Geometry: final body of the model. Coordinates: model frame, mm. A direction names the side the tool comes from. Coordinates: 2 decimals unless noted, no trailing zeros. Order: outer loops, then holes, each group sorted by start corner. A loop starts at its lowest first (then second) coordinate and runs counter-clockwise, first axis right, second up. Notation, with made-up numbers: (-18, 0) -> (32, 0) arc R29 cw to (32, 23) -> close; hole circle Ø10 at (9.5, 88). An arc over 180 degrees is marked (long way). Answer in a Markdown table with one row per item. Add a question column.
1) Section query A-A on x = 33. Return the cut outline in (y, z), then the cut area to 3 significant figures.
2) Section query B-B on y = 0. Return the cut outline in (x, z).
3) Set-up query: faces 4 (the face through (60.79, 13.61, 5.3)), 5 (the face through (-36.71, 28.26, 4.93)), 6 (the face through (-38.6, -1.9, 4.9)), 7 (the face through (-34.55, 8.38, 4.93)). Return all of +Z, -Z, +X, -X, +Y, -Y with unobstructed straight access to the full face (end or side cutting, diameter ignored); none if empty.
4) Ray query, line 1 (Y direction, x = 0, z = 7.75); line 2 (Y direction, x = 23.5, z = 0.5); line 3 (Y direction, x = -33.5, z = 1.75). Return the intervals inside material, ascending. Write a range as from..to.
5) Pull-direction query (Y, two-part tool) for faces 1 (the face through (-29.41, -92.26, 4.93)), 2 (the face through (11, -14, 0)), 3 (the face through (20.21, 23.37, 4.93)); classes: +Y half, -Y half, draft (parallel to the pull), parting line (faces both ways), or undercut.
6) Contact query for flat-ended pins moving along their axis: P1, Ø1.1, axis at x = 96, z = 7, coming from the -Y side; P2, Ø3, axis at y = -69, z = 6, coming from the +X side; P3, Ø3, axis at y = 17, z = 8, coming from the -X side. Output: stop coordinate, or through.
7) Section query D-D on z = 5.75. Count the separate pieces of the cut face and the enclosed holes in it, then the cut area to 3 significant figures.
8) Section query C-C on x = 0. Return the cut outline in (y, z).
```python
from build123d import *

# Parameters (mm, degrees)
SKETCH1_R           = 5.958520806
BOSS_EXTRUDE1_DEPTH = 10
SKETCH4_R           = 21.186821389
SKETCH4_R_2         = 2.5
CUT_EXTRUDE4_DEPTH  = 10
CUT_EXTRUDE5_DEPTH  = 24
SKETCH6_W           = 3.587503093
SKETCH6_H           = 10
CUT_EXTRUDE8_DEPTH  = 24
CUT_EXTRUDE9_DEPTH  = 24


with BuildPart() as part:
    # Sketch1 → Boss-Extrude1 (new body)
    with BuildSketch(Plane.XY):
        with BuildLine():
            Line((-43.641418847, 47.659934688), (-41.617733216, 27.762580681))
            Line((-41.617733216, 27.762580681), (-31.669056213, 28.774423496))
            Line((-31.669056213, 28.774423496), (-29.645370582, 8.877069489))
            Line((-29.645370582, 8.877069489), (-39.594047586, 7.865226674))
            Line((-39.594047586, 7.865226674), (-37.570361955, -12.032127333))
            Line((-37.570361955, -12.032127333), (-27.621684952, -11.020284517))
            Line((-27.621684952, -11.020284517), (-25.597999321, -30.917638524))
            Line((-25.597999321, -30.917638524), (-35.546676324, -31.929481339))
            Line((-35.546676324, -31.929481339), (-33.522990694, -51.826835346))
            Line((-33.522990694, -51.826835346), (-23.57431369, -50.814992531))
            Line((-23.57431369, -50.814992531), (-21.55062806, -70.712346537))
            Line((-21.55062806, -70.712346537), (-31.499305063, -71.724189353))
            Line((-31.499305063, -71.724189353), (-27.26172937, -113.389032166))
            Line((-27.26172937, -113.389032166), (95, -113.389032166))
            Line((95, -113.389032166), (95, 30.000000002))
            Line((95, 30.000000002), (98.587503094, 30.000000003))
            add(Edge.make_bspline(
                [(80, 47.659934688), (90.261106229, 39.851185476), (98.587503094, 30.000000003)],
                knots=[0, 0, 0, 1, 1, 1], degree=2))
            Line((80, 47.659934688), (-43.641418847, 47.659934688))
        make_face()
        Circle(SKETCH1_R, mode=Mode.SUBTRACT)
    extrude(amount=BOSS_EXTRUDE1_DEPTH)

    # Sketch4 → Cut-Extrude4 (cut)
    with BuildSketch(Plane(origin=(0, 0, 0), x_dir=(-1, 0, 0), z_dir=(0, 0, -1))):
        with Locations((-6.436847568, -67.192387913)):
            Circle(SKETCH4_R)
        with Locations((25.585650799, 21.365024531)):
            Circle(SKETCH4_R_2)
        with Locations((-21.365024531, 25.585650799)):
            Circle(SKETCH4_R_2)
        with Locations((14.627270614, -93.026333125)):
            Circle(SKETCH4_R_2)
        with Locations((-32.27079278, -88.256506094)):
            Circle(SKETCH4_R_2)
        with Locations((19.397097645, -46.128269731)):
            Circle(SKETCH4_R_2)
        with Locations((-27.500965749, -41.3584427)):
            Circle(SKETCH4_R_2)
        with Locations((-25.585650799, -21.365024531)):
            Circle(SKETCH4_R_2)
        with Locations((21.365024531, -25.585650799)):
            Circle(SKETCH4_R_2)
    extrude(amount=-CUT_EXTRUDE4_DEPTH, mode=Mode.SUBTRACT)

    # Sketch5 → Cut-Extrude5 (cut)
    with BuildSketch(Plane(origin=(-775.166388991, -380.154744581, 157.441443413), x_dir=(0.898957124, -0.049188488, -0.435266105), z_dir=(0.36537989, -0.463875199, 0.807042338))):
        Polygon((845.932415327, 510.73775684), (653.191404901, 500.019526219), (653.191404901, 468.74716356), (845.932415327, 468.74716356), align=None)
    extrude(amount=CUT_EXTRUDE5_DEPTH, mode=Mode.SUBTRACT)

    # Sketch6 → Cut-Extrude8 (cut)
    with BuildSketch(Plane.XZ.offset(-29.999999993)):
        with Locations((96.79375155, 5)):
            Rectangle(SKETCH6_W, SKETCH6_H)
        Polygon((71.218728104, 10), (93.306488259, 0), (95.000000003, 0), (95.000000003, 10), align=None)
    extrude(amount=CUT_EXTRUDE8_DEPTH, mode=Mode.SUBTRACT)

    # Sketch7 → Cut-Extrude9 (cut)
    with BuildSketch(Plane.XY.offset(10)):
        Polygon((95, -113.389032166), (49.555056821, -113.389032166), (49.555056821, -4.461625106), (95, 0), align=None)
    extrude(amount=-CUT_EXTRUDE9_DEPTH, mode=Mode.SUBTRACT)


solid = part.part
```
Result:
| question | item | result |
|---|---|---|
| 1 | outline | (-113.39, 0) -> (-90.65, 0) -> (-90.65, 10) -> (-113.39, 10) -> close; (-85.87, 0) -> (47.66, 0) -> (47.66, 10) -> (-0.1, 10) -> (-3.56, 8.02) -> (-4.45, 10) -> (-85.87, 10) -> close |
| 1 | area | 1,560 mm2 |
| 2 | outline | (-38.79, 0) -> (-5.96, 0) -> (-5.96, 10) -> (-38.79, 10) -> close; (5.96, 0) -> (55.22, 0) -> (33.13, 10) -> (5.96, 10) -> close |
| 3 | face 4 | +Z, +X |
| 3 | face 5 | +Z, -Z |
| 3 | face 6 | +Z, -Z, -X, -Y |
| 3 | face 7 | +Z, -Z, -X |
| 4 | line 1 | -113.39..-87.38, -47.01..-5.96, 5.96..47.66 |
| 4 | line 2 | -113.39..-79.75, -54.63..-22.74, -19.99..24.28, 26.89..47.66 |
| 4 | line 3 | -51.82..-31.72, -11.62..8.49, 28.59..47.66 |
| 5 | face 1 | -Y half |
| 5 | face 2 | draft |
| 5 | face 3 | undercut |
| 6 | P1 | y = 30 |
| 6 | P2 | x = 49.56 |
| 6 | P3 | x = -30.62 |
| 7 | separate pieces | 1 |
| 7 | enclosed holes | 10 |
| 7 | area | 12,400 mm2 |
| 8 | outline | (-113.39, 0) -> (-87.38, 0) -> (-87.38, 10) -> (-113.39, 10) -> close; (-47.01, 0) -> (-5.96, 0) -> (-5.96, 10) -> (-47.01, 10) -> close; (5.96, 0) -> (47.66, 0) -> (47.66, 10) -> (5.96, 10) -> close |
